Input: part model. Units: mm. Frame: model coordinates. A direction names the side the tool comes from. Give positions to 0.01 mm unless a question says otherwise; leave off trailing zeros. Loops run counter-clockwise (first coordinate to the right, second up) from the corner with the lowest first, then second, coordinate; pieces in that order, holes last.
from build123d import *

# Parameters (mm, degrees)
BOSS_EXTRUDE1_DEPTH = 87
SKETCH2_R           = 2.25
BOSS_EXTRUDE2_DEPTH = 7
BOSS_EXTRUDE3_DEPTH = 22


with BuildPart() as part:
    # Sketch1 → Boss-Extrude1 (new body)
    with BuildSketch(Plane.XY):
        with BuildLine():
            Line((0, 0), (32.5, 0))
            add(Edge.make_bspline(
                [(32.5, 60.3), (60.3, 30.15), (32.5, 0)],
                knots=[0, 0, 0, 1, 1, 1], degree=2))
            Line((32.5, 60.3), (0, 60.3))
            add(Edge.make_bspline(
                [(0, 60.3), (-27.8, 30.15), (0, 0)],
                knots=[0, 0, 0, 1, 1, 1], degree=2))
        make_face()
    extrude(amount=BOSS_EXTRUDE1_DEPTH)

    # Sketch2 → Boss-Extrude2 (add)
    with BuildSketch(Plane.XY.offset(87)):
        with BuildLine():
            Line((-13.9, 55.3), (-13.9, 5))
            ThreePointArc((-13.9, 5), (-12.435533906, 1.464466094), (-8.9, 0))
            Line((-8.9, 0), (41.4, 0))
            ThreePointArc((41.4, 0), (44.935533906, 1.464466094), (46.4, 5))
            Line((46.4, 5), (46.4, 55.3))
            ThreePointArc((46.4, 55.3), (44.935533906, 58.835533906), (41.4, 60.3))
            Line((41.4, 60.3), (-8.9, 60.3))
            ThreePointArc((-8.9, 60.3), (-12.435533906, 58.835533906), (-13.9, 55.3))
        make_face()
        with Locations((40.998737342, 54.898737342)):
            Circle(SKETCH2_R, mode=Mode.SUBTRACT)
        with Locations((40.998737342, 5.401262658)):
            Circle(SKETCH2_R, mode=Mode.SUBTRACT)
        with Locations((-8.498737342, 5.401262658)):
            Circle(SKETCH2_R, mode=Mode.SUBTRACT)
        with Locations((-8.498737342, 54.898737342)):
            Circle(SKETCH2_R, mode=Mode.SUBTRACT)
    extrude(amount=BOSS_EXTRUDE2_DEPTH)

    # Sketch3 → Boss-Extrude3 (add)
    with BuildSketch(Plane.XY.offset(94)):
        with BuildLine():
            Line((18.300133509, 33.585203779), (14.300133509, 33.585203779))
            ThreePointArc((14.300133509, 33.585203779), (13.489384054, 27.339250545), (19.735337287, 28.15))
            Line((19.735337287, 28.15), (19.735337287, 32.15))
            ThreePointArc((19.735337287, 32.15), (19.110882964, 32.960749455), (18.300133509, 33.585203779))
        make_face()
    extrude(amount=BOSS_EXTRUDE3_DEPTH)


solid = part.part
(1) Mould query, pull axis Y, two halves, no side actions, for faces 6 (the cylindrical face through (40.71, 57.13, 90.45)), 7 (the cylindrical face through (-12.4, 58.87, 90.45)), 8 (the flat face through (-11, 10, 87)). Classes: +Y half, -Y half, draft (parallel to the pull), parting line (faces both ways), or undercut.
Values follow:
face 6: undercut
face 7: +Y half
face 8: draft
(2) Cut plane B-B (x = 17). Return the cut outline in (y, z), and give its area (3 significant figures).
Values follow:
outline: (0, 0) - (60.3, 0) - (60.3, 94) - (33.59, 94) - (33.59, 116) - (26.24, 116) - (26.24, 94) - (0, 94) - close
area: 5,830 mm2
(3) Ray query, probe 1 along Z at (x, y) = (22, 25); probe 2 along X at (y, z) = (29.5, 76); probe 3 along X at (y, z) = (18, 7). Return the intervals inside material, ascending.
Values follow:
probe 1: z = 0 to 94
probe 2: x = -13.89 to 46.39
probe 3: x = -11.64 to 44.14
(4) Cut plane C-C (z = 106). Return the cut outline in (x, y) (3 decimals), and give its area (3 significant figures).
Values follow:
outline: (14.3, 33.585) arc R3.975 ccw (long way) to (19.735, 28.15) - (19.735, 32.15) arc R3.975 ccw to (18.3, 33.585) - close
area: 46.7 mm2
(5) Cut plane A-A (z = 91). Return the cut outline in (x, y).
Values follow:
outline: (-13.9, 5) arc R5 ccw to (-8.9, 0) - (41.4, 0) arc R5 ccw to (46.4, 5) - (46.4, 55.3) arc R5 ccw to (41.4, 60.3) - (-8.9, 60.3) arc R5 ccw to (-13.9, 55.3) - close; hole circle Ø4.5 at (-8.5, 5.4); hole circle Ø4.5 at (-8.5, 54.9); hole circle Ø4.5 at (41, 5.4); hole circle Ø4.5 at (41, 54.9)
(6) Pin query (flat end, axial travel): pin 1 Ø4 at (x, y) = (-3.5, 48.5) entering from -Z; pin 2 Ø3.5 at (x, y) = (-8.5, 54.9) entering from +Z; pin 3 Ø3 at (x, z) = (17, 104) entering from +Y; pin 4 Ø3 at (y, z) = (35, 79.5) entering from +X. Return the tip coordinate at first contact, or that it passes through.
Values follow:
pin 1: stops at z = 0
pin 2: passes through
pin 3: stops at y = 33.59
pin 4: stops at x = 46.23
(7) Reachability of faces 1 (the flat face through (16, 33.585, 105)), 2 (the flat face through (19.735, 30, 105)), 3 (the cylindrical face through (-12.47, 1.5, 90.45)), 4 (the flat face through (42, 8, 87)), 5 (the flat face through (-10, 52, 87)) from +Z, -Z, +X, -X, +Y, -Y: full face, straight path, thin tool, end or side. Return the list, or none.
Values follow:
face 1: +Z, +X, -X, +Y
face 2: +Z, +X, +Y, -Y
face 3: +Z, -Z, -X, -Y
face 4: -Z, +X, -Y
face 5: -Z, -X, +Y
